Design review of the part built by this model. Coordinates are the model's own, in mm. Face numbers are marked on the shaded views. A direction names the side the tool comes from. Give positions to 0.01 mm unless a question says otherwise; leave off trailing zeros. Order: outer loops, then holes, each group sorted by start corner. A loop starts at its lowest first (then second) coordinate and runs counter-clockwise, first axis right, second up. Notation, with made-up numbers: (52, 18) -> (76, 18) arc R16 cw to (76, 39) -> close; hole circle Ø1 at (28, -20). An arc over 180 degrees is marked (long way). Return JSON: item names as keys, results as strings.
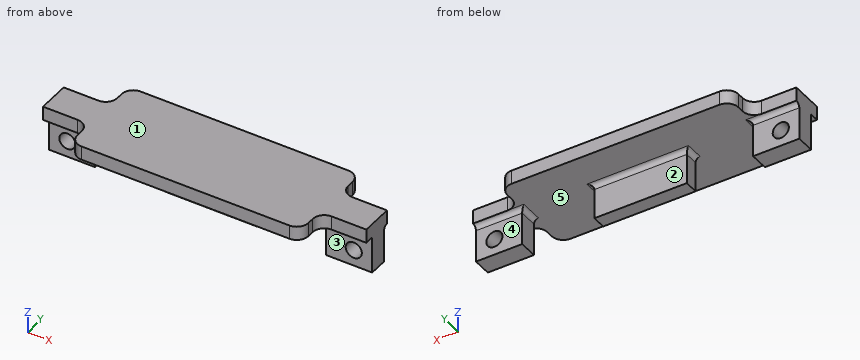
```python
from build123d import *

# Parameters (mm, degrees)
SKETCH1_W           = 20
SKETCH1_H           = 155
BOSS_EXTRUDE1_DEPTH = 4
SKETCH2_W           = 20
SKETCH2_H           = 4
BOSS_EXTRUDE3_DEPTH = 50
RIB2_REACH          = 96.986
SKETCH7_WALL_W      = 290.205463948
SKETCH7_WALL_H      = 4
SKETCH8_W           = 20
SKETCH8_H           = 3
BOSS_EXTRUDE4_DEPTH = 3.5
SKETCH9_W           = 70
SKETCH9_H           = 5
BOSS_EXTRUDE6_DEPTH = 3
SKETCH10_W          = 10
SKETCH10_H          = 4
BOSS_EXTRUDE7_DEPTH = 8
SKETCH12_R          = 1.75
CUT_EXTRUDE1_DEPTH  = 10
SKETCH13_W          = 111.319070758
SKETCH13_H          = 99.743885808
CUT_EXTRUDE2_DEPTH  = 152
SKETCH14_W          = 50
SKETCH14_H          = 3
BOSS_EXTRUDE8_DEPTH = 6.5
FILLET1_R           = 1
FILLET2_R           = 2.5


with BuildPart() as part:
    # Sketch1 → Boss-Extrude1 (new body)
    with BuildSketch(Plane.XY):
        Rectangle(SKETCH1_W, SKETCH1_H)
    extrude(amount=BOSS_EXTRUDE1_DEPTH)

    # Sketch2 → Boss-Extrude3 (add)
    with BuildSketch(Plane.XY.offset(4)):
        with Locations((0, -75.5)):
            Rectangle(SKETCH2_W, SKETCH2_H)
    extrude(amount=BOSS_EXTRUDE3_DEPTH)

    # Sketch7 wall → Rib2 (add, up to next)
    with BuildSketch(Plane(origin=(0, -26, 16.5), x_dir=(0, 0.967074537263, -0.25449329928), z_dir=(0, 0.25449329928, 0.967074537263)), mode=Mode.PRIVATE) as rib2_sk1:
        Rectangle(SKETCH7_WALL_W, SKETCH7_WALL_H)
    rib2_tool1 = extrude(rib2_sk1.sketch, amount=-RIB2_REACH, mode=Mode.PRIVATE) - part.part
    add(rib2_tool1.solids().sort_by_distance((0, -26, 16.5))[0])

    # Sketch8 → Boss-Extrude4 (add)
    with BuildSketch(Plane.XY.offset(4)):
        with Locations((0, 76)):
            Rectangle(SKETCH8_W, SKETCH8_H)
    extrude(amount=BOSS_EXTRUDE4_DEPTH)

    # Sketch9 → Boss-Extrude6 (add)
    with BuildSketch(Plane.XY.offset(7.5)):
        with Locations((0, 77)):
            Rectangle(SKETCH9_W, SKETCH9_H)
    boss_extrude6 = extrude(amount=BOSS_EXTRUDE6_DEPTH)

    # Sketch10 → Boss-Extrude7 (add)
    with BuildSketch(Plane(origin=(0, 0, 7.5), x_dir=(-1, 0, 0), z_dir=(0, 0, -1))):
        with Locations((30, 76.5)):
            Rectangle(SKETCH10_W, SKETCH10_H)
        with Locations((-30, 76.5)):
            Rectangle(SKETCH10_W, SKETCH10_H)
    extrude(amount=BOSS_EXTRUDE7_DEPTH)

    # Sketch12 → Cut-Extrude1 (cut)
    with BuildSketch(Plane(origin=(0, 78.5, 0), x_dir=(1, 0, 0), z_dir=(0, 1, 0))):
        with Locations(Location((-31, -3, 0), (0, 0, 270))):
            Circle(SKETCH12_R)
        with Locations(Location((31, -3, 0), (0, 0, 270))):
            Circle(SKETCH12_R)
    extrude(amount=-CUT_EXTRUDE1_DEPTH, mode=Mode.SUBTRACT)

    # Sketch13 → Cut-Extrude2 (cut)
    with BuildSketch(Plane.XZ.offset(77.5)):
        with Locations((2.652852139, 20.474703111)):
            Rectangle(SKETCH13_W, SKETCH13_H)
    extrude(amount=-CUT_EXTRUDE2_DEPTH, mode=Mode.SUBTRACT)

    # Sketch14 → Boss-Extrude8 (add)
    with BuildSketch(Plane(origin=(0, 79.5, 0), x_dir=(1, 0, 0), z_dir=(0, 1, 0))):
        with Locations((0, -9)):
            Rectangle(SKETCH14_W, SKETCH14_H)
    boss_extrude8 = extrude(amount=BOSS_EXTRUDE8_DEPTH)

    # Mirror1: Boss-Extrude6, Boss-Extrude8 across plane
    add(boss_extrude6.mirror(Plane(origin=(0, 76, 0), x_dir=(0, 0, 1), z_dir=(0, -1, 0))))
    add(boss_extrude8.mirror(Plane(origin=(0, 76, 0), x_dir=(0, 0, 1), z_dir=(0, -1, 0))))

    # Fillet1
    fillet1_edges = [part.edges().sort_by_distance(p)[0] for p in [
        (10, 76, 7.5),
        (0, 77.5, 7.5),
        (-10, 76, 7.5),
        (-30, 78.5, 7.5),
        (-25, 76.5, 7.5),
        (25, 76.5, 7.5),
        (30, 78.5, 7.5),
    ]]
    fillet(fillet1_edges, radius=FILLET1_R - 0.0001)  # a hair under: the kernel refuses the full size

    # Fillet2
    fillet2_edges = [part.edges().sort_by_distance(p)[0] for p in [
        (-25, 79.5, 9),
        (25, 79.5, 9),
        (-25, 86, 9),
        (25, 86, 9),
        (-25, 66, 9),
        (25, 66, 9),
        (-25, 72.5, 9),
        (25, 72.5, 9),
    ]]
    fillet(fillet2_edges, radius=FILLET2_R)


solid = part.part
```
Item 1: Add section D-D (x = -7). Give the boundary of the cut face in (y, z).
Result set:
{"outline": "(66, 7.5) -> (74.5, 7.5) -> (74.5, 0) -> (77.5, 0) -> (77.5, 6.5) arc R1 cw to (78.5, 7.5) -> (86, 7.5) -> (86, 10.5) -> (66, 10.5) -> close"}
Item 2: For pin 1 (0.8 mm diameter, centred on y = 83, z = 9.5, fed in from +X); pin 2 (2.5 mm diameter, centred on x = 32, z = 9, fed in from +Y); pin 3 (0.8 mm diameter, centred on y = 83, z = 9, fed in from -X); pin 4 (1 mm diameter, centred on x = -12, z = 5.5, fed in from -Y) (3 decimals), all flat-tipped, find the tip position at first contact; note any pin that passes through.
Result set:
{"pin 1": "stops at x = 25", "pin 2": "stops at y = 79.5", "pin 3": "stops at x = -25", "pin 4": "passes through"}
Item 3: Add section C-C (y = 75.5). Give the boundary of the cut face in (x, z), plus the area to 3 significant figures.
Result set:
{"outline": "(-35, -0.5) -> (-25, -0.5) -> (-25, 6.5) arc R1 cw to (-24, 7.5) -> (-11, 7.5) arc R1 cw to (-10, 6.5) -> (-10, 0) -> (10, 0) -> (10, 6.5) arc R1 cw to (11, 7.5) -> (24, 7.5) arc R1 cw to (25, 6.5) -> (25, -0.5) -> (35, -0.5) -> (35, 10.5) -> (-35, 10.5) -> close; hole circle Ø3.5 at (-31, 3); hole circle Ø3.5 at (31, 3)", "area": "502 mm^2"}
Item 4: Machinability: for the marked faces 3, 4 and 5, which of the approach directions +Z, -Z, +X, -X, +Y, -Y give a long, thin tool a straight path to every point of the face, cutting with its end or side? Answer none if there is none.
Result set:
{"face 3": "-Z, +X, -X, -Y", "face 4": "-Z, +X, -X, +Y", "face 5": "-Z"}
Item 5: Add section A-A (z = 3). Give the boundary of the cut face in (x, y), plus the area to 3 significant figures.
Result set:
{"outline": "(-35, 74.5) -> (-32.75, 74.5) -> (-32.75, 78.5) -> (-35, 78.5) -> close; (-29.25, 74.5) -> (-25, 74.5) -> (-25, 78.5) -> (-29.25, 78.5) -> close; (-10, 74.5) -> (10, 74.5) -> (10, 77.5) -> (-10, 77.5) -> close; (25, 74.5) -> (29.25, 74.5) -> (29.25, 78.5) -> (25, 78.5) -> close; (32.75, 74.5) -> (35, 74.5) -> (35, 78.5) -> (32.75, 78.5) -> close", "area": "112 mm^2"}
Item 6: Wall thickness on L1, parallel to X at y = 76.6, z = 3; L2, parallel to X at y = 76.5, z = 1.5; L3, parallel to Z at x = -24.5, y = 84: over which ranges is each line inside the solid? List them lowest first. Write a range as [from, to].
Result set:
{"L1": "x = [-35, -32.75], [-29.25, -25], [-10, 10], [25, 29.25], [32.75, 35]", "L2": "x = [-35, -31.9], [-30.1, -25], [-10, 10], [25, 30.1], [31.9, 35]", "L3": "z = [7.5, 10.5]"}
Item 7: Mouldability with a two-part tool opening along X and no side actions: class the marked faces 1 and 2 as released by +X, released by -X, zero draft, split by the parting line, or undercut.
Result set:
{"face 1": "zero draft", "face 2": "undercut"}
